Read the model definition and answer for the solid it produces. Units are mm, in the model's axes. A direction names the side the tool comes from. Coordinates: 2 decimals unless noted, no trailing zeros. Loops run counter-clockwise (first coordinate to the right, second up) from the corner with the lowest first, then second, coordinate; pieces in that order, holes last. Notation, with made-up numbers: (-40, 21.25) -> (-33, 21.25) arc R7 cw to (-33, 27.25) -> close; hole circle Ø4 at (-27.75, 69.25). An arc over 180 degrees is marked (long way). Answer as a JSON object with one key per item and string values. Group by question number.
Q1. The part is cut by section B-B on y = 98. Write down the section's boundary in (x, z), and give its area (3 significant figures).
Q2. Straight lines are drawn through the part: line 1 along X through (y, z) = (108.5, 0); line 2 along X through (y, z) = (110.25, 0). For each, find the intervals that lie inside material, in ascending order. Write a range as [from, to].
Q3. Each of these flat-tipped pins is pushed along its axis until it touches: P1, Ø8, axis at y = 76, z = -15, coming from the +X side; P2, Ø6, axis at y = 29, z = 5, coming from the -X side; P3, Ø8, axis at y = 76, z = -14.5, coming from the -X side; P4, Ø12, axis at x = 0, z = 0, coming from the +Y side. Where does it stop, or does it pass through?
Q4. Determine the mould class of faces 1 (the flat face through (38.366, 0.986, 39.916)), 2 (the flat face through (6.2, 111, 0)), 3 (the flat face through (11, 2, -20)) for opening direction Z: released by +Z, released by -Z, zero draft, split by the parting line, or undercut.
Q5. For faces 4 (the cylindrical face through (7.429, 107.437, 5.697)), 5 (the flat face through (-38.134, 0.986, 40.084)), determine the directions among +Z, -Z, +X, -X, +Y, -Y from which every point of the face is accessible in a straight line to the end or side of a thin tool.
Q6. The part is cut by section D-D on x = 39.5. Write down the section's boundary in (y, z), and give its area (3 significant figures).
Q7. The part is cut by section C-C on y = 14. Write down the section's boundary in (x, z), and give its area (3 significant figures).
from build123d import *

# Parameters (mm, degrees)
F1_DEPTH = 2
F6_DEPTH = 3


with BuildPart() as f1:
    # F0 (on Front) → F1 (new body)
    with BuildSketch(Plane.XZ):
        Polygon((-52.5, -46), (52.5, -46), (46.5, 34), (30, 46), (-30, 46), (-46.5, 34), align=None)
    extrude(amount=-F1_DEPTH)

    # F2 (on Top) → F3 (revolve, cut)
    with BuildSketch(Plane.XY):
        Polygon((-20, 0), (0, 0), (0, 103), (-7.3619631902, 103), align=None)
    revolve(axis=Axis((0, 81.5, 0), (0, -1, 0)), mode=Mode.SUBTRACT)

    # F2 (on Top) → F4 (revolve)
    with BuildSketch(Plane.XY):
        Polygon((-22, 0), (-20, 0), (-7.3619631902, 103), (-9.3619631902, 103), align=None)
        Polygon((-9.3619631902, 103), (-7.3619631902, 103), (-7.3619631902, 112), (-8.2576687117, 112), align=None)
        Polygon((-9.3619631902, 112), (-9.3619631902, 103), (-8.2576687117, 112), align=None)
    revolve(axis=Axis((0, 2, 0), (0, -1, 0)))

    # F5 (on face) → F6 (join)
    with BuildSketch(Plane(origin=(0, 112, 0), x_dir=(-1, 0, 0), z_dir=(0, 1, 0))):
        with BuildLine():
            Line((-6.2, -3.9696979751), (-6.2, 0))
            Line((-6.2, 0), (-6.2, 3.9696979751))
            ThreePointArc((-6.2, 3.9696979751), (-7.3619631902, 0), (-6.2, -3.9696979751))
        make_face()
        with BuildLine():
            Line((6.0885886352, 4.1385493165), (6.2, 0))
            Line((6.2, 0), (6.3024315003, -3.8049782124))
            ThreePointArc((6.3024315003, -3.8049782124), (7.0921354587, -1.9748712995), (7.3619631902, 0))
            ThreePointArc((7.3619631902, 0), (7.0364219397, 2.1650100001), (6.0885886352, 4.1385493165))
        make_face()
    extrude(amount=-F6_DEPTH)


solid = f1.part
Final values:
{
 "1": {"outline": "circle Ø19.95 at (0, 0); hole circle Ø15.95 at (0, 0)", "area": "113 mm2"},
 "2": {"line 1": "x = [-9.36, -7.36], [7.36, 9.36]", "line 2": "x = [-9.36, -6.2], [6.2, 9.36]"},
 "3": {"P1": "stops at x = 6.37", "P2": "stops at x = -18.48", "P3": "stops at x = -7.16", "P4": "passes through"},
 "4": {"face 1": "released by +Z", "face 2": "undercut", "face 3": "zero draft"},
 "5": {"face 4": "+Y", "face 5": "+Z, -X, +Y, -Y"},
 "6": {"outline": "(0, -46) -> (2, -46) -> (2, 39.09) -> (0, 39.09) -> close", "area": "170 mm2"},
 "7": {"outline": "circle Ø40.56 at (0, 0); hole circle Ø36.56 at (0, 0)", "area": "242 mm2"}
}
